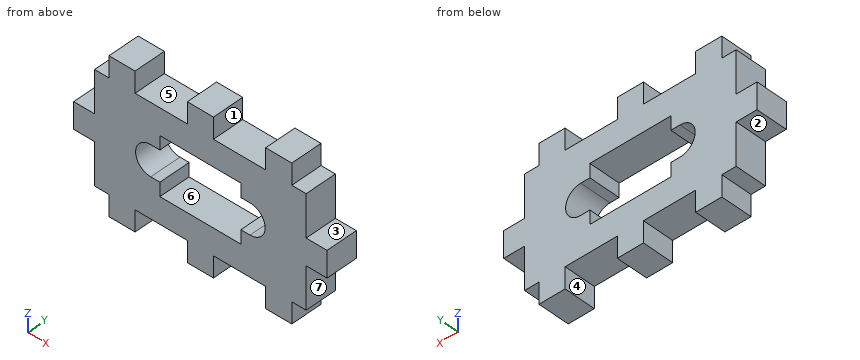
```python
from build123d import *

# Parameters (mm, degrees)
SKETCH1_W           = 15.5
SKETCH1_H           = 11
BOSS_EXTRUDE1_DEPTH = 1.6
BOSS_EXTRUDE2_DEPTH = 1.6
SKETCH3_W           = 40.5
SKETCH3_H           = 21
BOSS_EXTRUDE3_DEPTH = 6
CUT_EXTRUDE1_DEPTH  = 2.6
SKETCH5_W           = 5
SKETCH5_H           = 4
BOSS_EXTRUDE4_DEPTH = 6
LPATTERN1_COUNT     = 2
LPATTERN1_PITCH     = 15
LPATTERN1_COL_COUNT = 2
LPATTERN1_COL_PITCH = 15
SKETCH6_W           = 4
SKETCH6_H           = 5
BOSS_EXTRUDE5_DEPTH = 6


with BuildPart() as part:
    # Sketch1 → Boss-Extrude1 (new body)
    with BuildSketch(Plane(origin=(0, 0, 0), x_dir=(1, 0, 0), z_dir=(0, 1, 0))):
        with Locations((7.75, -5.5)):
            Rectangle(SKETCH1_W, SKETCH1_H)
    extrude(amount=BOSS_EXTRUDE1_DEPTH)

    # Sketch2 → Boss-Extrude2 (add, through all)
    with BuildSketch(Plane(origin=(0, 1.6, 0), x_dir=(1, 0, 0), z_dir=(0, 1, 0))):
        with BuildLine():
            Line((-1.75, -4), (-1.75, -2.6))
            ThreePointArc((-1.75, -2.6), (-4.65, -5.5), (-1.75, -8.4))
            Line((-1.75, -8.4), (-1.75, -7))
            ThreePointArc((-1.75, -7), (-3.25, -5.5), (-1.75, -4))
        make_face()
        with BuildLine():
            ThreePointArc((0, -3.187533784), (-0.827002716, -2.750804479), (-1.75, -2.6))
            Line((-1.75, -2.6), (-1.75, -4))
            ThreePointArc((-1.75, -4), (-0.689339828, -4.439339828), (-0.25, -5.5))
            ThreePointArc((-0.25, -5.5), (-0.689339828, -6.560660172), (-1.75, -7))
            Line((-1.75, -7), (-1.75, -8.4))
            ThreePointArc((-1.75, -8.4), (-0.827002716, -8.249195521), (0, -7.812466216))
            Line((0, -7.812466216), (0, -3.187533784))
        make_face()
        with BuildLine():
            Line((0, -2.6), (-1.75, -2.6))
            ThreePointArc((-1.75, -2.6), (-0.827002716, -2.750804479), (0, -3.187533784))
            Line((0, -3.187533784), (0, -2.6))
        make_face()
        with BuildLine():
            ThreePointArc((0, -7.812466216), (-0.827002716, -8.249195521), (-1.75, -8.4))
            Line((-1.75, -8.4), (0, -8.4))
            Line((0, -8.4), (0, -7.812466216))
        make_face()
        with BuildLine():
            ThreePointArc((20.15, -5.5), (19.300609665, -3.449390335), (17.25, -2.6))
            Line((17.25, -2.6), (17.25, -4))
            ThreePointArc((17.25, -4), (18.310660172, -4.439339828), (18.75, -5.5))
            ThreePointArc((18.75, -5.5), (18.310660172, -6.560660172), (17.25, -7))
            Line((17.25, -7), (17.25, -8.4))
            ThreePointArc((17.25, -8.4), (19.300609665, -7.550609665), (20.15, -5.5))
        make_face()
        with BuildLine():
            Line((17.25, -4), (17.25, -2.6))
            ThreePointArc((17.25, -2.6), (16.327002716, -2.750804479), (15.5, -3.187533784))
            Line((15.5, -3.187533784), (15.5, -7.812466216))
            ThreePointArc((15.5, -7.812466216), (16.327002716, -8.249195521), (17.25, -8.4))
            Line((17.25, -8.4), (17.25, -7))
            ThreePointArc((17.25, -7), (15.75, -5.5), (17.25, -4))
        make_face()
        with BuildLine():
            Line((17.25, -2.6), (15.5, -2.6))
            Line((15.5, -2.6), (15.5, -3.187533784))
            ThreePointArc((15.5, -3.187533784), (16.327002716, -2.750804479), (17.25, -2.6))
        make_face()
        with BuildLine():
            Line((15.5, -7.812466216), (15.5, -8.4))
            Line((15.5, -8.4), (17.25, -8.4))
            ThreePointArc((17.25, -8.4), (16.327002716, -8.249195521), (15.5, -7.812466216))
        make_face()
    extrude(amount=-BOSS_EXTRUDE2_DEPTH)

    # Sketch4 → Cut-Extrude1 (cut, through all)
    with BuildSketch(Plane(origin=(0, 1.6, 0), x_dir=(1, 0, 0), z_dir=(0, 1, 0))):
        with BuildLine():
            Line((0, 0), (0, -2.6))
            Line((0, -2.6), (-1.75, -2.6))
            ThreePointArc((-1.75, -2.6), (-4.65, -5.5), (-1.75, -8.4))
            Line((-1.75, -8.4), (0, -8.4))
            Line((0, -8.4), (0, -11))
            Line((0, -11), (15.5, -11))
            Line((15.5, -11), (15.5, -8.4))
            Line((15.5, -8.4), (17.25, -8.4))
            ThreePointArc((17.25, -8.4), (20.15, -5.5), (17.25, -2.6))
            Line((17.25, -2.6), (15.5, -2.6))
            Line((15.5, -2.6), (15.5, 0))
            Line((15.5, 0), (0, 0))
        make_face()
    extrude(amount=-CUT_EXTRUDE1_DEPTH, mode=Mode.SUBTRACT)


with BuildPart() as body_2:
    # Sketch3 → Boss-Extrude3 (new body)
    with BuildSketch(Plane(origin=(0, 1.6, 0), x_dir=(1, 0, 0), z_dir=(0, 1, 0))):
        with Locations((7.75, -5.5)):
            Rectangle(SKETCH3_W, SKETCH3_H)
        with BuildLine():
            Line((0, 0), (0, -2.6))
            Line((0, -2.6), (-1.75, -2.6))
            ThreePointArc((-1.75, -2.6), (-4.65, -5.5), (-1.75, -8.4))
            Line((-1.75, -8.4), (0, -8.4))
            Line((0, -8.4), (0, -11))
            Line((0, -11), (15.5, -11))
            Line((15.5, -11), (15.5, -8.4))
            Line((15.5, -8.4), (17.25, -8.4))
            ThreePointArc((17.25, -8.4), (20.15, -5.5), (17.25, -2.6))
            Line((17.25, -2.6), (15.5, -2.6))
            Line((15.5, -2.6), (15.5, 0))
            Line((15.5, 0), (0, 0))
        make_face(mode=Mode.SUBTRACT)
    extrude(amount=BOSS_EXTRUDE3_DEPTH)

    # Sketch5 → Boss-Extrude4 (add, through all)
    with BuildSketch(Plane(origin=(0, 7.6, 0), x_dir=(1, 0, 0), z_dir=(0, 1, 0))):
        with Locations((7.75, 7)):
            Rectangle(SKETCH5_W, SKETCH5_H)
        with Locations((7.75, -18)):
            Rectangle(SKETCH5_W, SKETCH5_H)
    boss_extrude4 = extrude(amount=-BOSS_EXTRUDE4_DEPTH)

    # LPattern1: Boss-Extrude4 ×2
    with Locations(*[(i * LPATTERN1_PITCH, 0, 0) for i in range(1, LPATTERN1_COUNT)]):
        add(boss_extrude4)

    # LPattern1 col: Boss-Extrude4 ×2
    with Locations(*[(-i * LPATTERN1_COL_PITCH, 0, 0) for i in range(1, LPATTERN1_COL_COUNT)]):
        add(boss_extrude4)

    # Sketch6 → Boss-Extrude5 (add, through all)
    with BuildSketch(Plane(origin=(0, 7.6, 0), x_dir=(1, 0, 0), z_dir=(0, 1, 0))):
        with Locations((-14.5, -5.5)):
            Rectangle(SKETCH6_W, SKETCH6_H)
        with Locations((30, -5.5)):
            Rectangle(SKETCH6_W, SKETCH6_H)
    extrude(amount=-BOSS_EXTRUDE5_DEPTH)


solid = body_2.part
```
Design review of the part built by this model. Coordinates are the model's own, in mm. Face numbers are marked on the shaded views. A direction names the side the tool comes from. Round coordinates to 2 decimals unless told otherwise and drop trailing zeros. Write each loop counter-clockwise with the first axis right and the second up, starting at its lowest first coordinate (ties: lowest second). Pieces come first, ordered by that corner, then holes. Notation, with made-up numbers: (-28.75, 27) -> (-21.75, 27) arc R7 cw to (-21.75, 33) -> close; hole circle Ø5 at (79.5, -25.5). An arc over 180 degrees is marked (long way). Write item = value, one per line. Start each with the question number.
1) Take a section at C-C, the plane z = 14.5. State the section outline as (x, y) points.
2) Tool access review of the marked faces 1, 2, 3 and 4: name each direction out of +Z, -Z, +X, -X, +Y, -Y from which nothing blocks a thin tool from reaching the whole face with its end or side.
3) Take a section at A-A, the plane z = 5.5. State the section outline as (x, y) points.
4) Wall thickness on probe 1 along X at (y, z) = (6.7, -5.75); probe 2 along Z at (x, y) = (1, 2.45); probe 3 along X at (y, z) = (2.3, 10.75): over which ranges is each line inside the solid? List them lowest first. Write a range as from..to.
5) Mouldability with a two-part tool opening along Z and no side actions: class the marked faces 5, 6 and 7 as +Z half, -Z half, draft (parallel to the pull), parting line (faces both ways), or undercut.
6) Take a section at B-B, the plane x = 3. State the section outline as (y, z) points.
7) Clearance check with flat-ended pins moving along their axes: pin 1 (3 mm diameter, centred on x = 4.5, y = 5.5, fed in from -Z); pin 2 (3 mm diameter, centred on y = 5, z = -6, fed in from +X); pin 3 (1.2 mm diameter, centred on y = 3, z = 18, fed in from +X); pin 4 (1.5 mm diameter, centred on y = 5.5, z = 9, fed in from -X). State where each tip first meets the part, or that it passes through.
Results list:
q1.outline = (-12.5, 1.6) -> (28, 1.6) -> (28, 7.6) -> (-12.5, 7.6) -> close
q2.face_1 = +Z, +Y, -Y
q2.face_2 = -Z, -X, +Y, -Y
q2.face_3 = +Z, +X, +Y, -Y
q2.face_4 = -Z, +Y, -Y
q3.outline = (-16.5, 1.6) -> (-4.65, 1.6) -> (-4.65, 7.6) -> (-16.5, 7.6) -> close; (20.15, 1.6) -> (32, 1.6) -> (32, 7.6) -> (20.15, 7.6) -> close
q4.probe_1 = -9.75..-4.75, 5.25..10.25, 20.25..25.25
q4.probe_2 = -5..0, 11..16
q4.probe_3 = -12.5..0, 15.5..28
q5.face_5 = +Z half
q5.face_6 = undercut
q5.face_7 = draft
q6.outline = (1.6, -5) -> (7.6, -5) -> (7.6, 0) -> (1.6, 0) -> close; (1.6, 11) -> (7.6, 11) -> (7.6, 16) -> (1.6, 16) -> close
q7.pin_1 = -9
q7.pin_2 = 28
q7.pin_3 = 25.25
q7.pin_4 = -12.5
